```python
from build123d import *
from build123d.topology import SkipClean

# Parameters (mm, degrees)
SKETCH3_R                = 15.9
BOSS_EXTRUDE1_DEPTH      = 35
SKETCH4_R                = 5
BOSS_EXTRUDE2_DEPTH      = 32.5
SKETCH7_W                = 4.2
SKETCH7_H                = 5.15
SKETCH7_W_2              = 5.6
SKETCH7_H_2              = 2.4
BOSS_EXTRUDE3_DEPTH      = 5
BOSS_EXTRUDE3_DEPTH_BACK = 5
SKETCH8_R                = 6.25
SKETCH8_R_2              = 3
SKETCH9_R                = 3
CUT_EXTRUDE1_DEPTH       = 16


with BuildPart() as part:
    # Sketch3 → Boss-Extrude1 (new body)
    with BuildSketch(Plane.XY):
        Circle(SKETCH3_R)
    extrude(amount=BOSS_EXTRUDE1_DEPTH)

    # Sketch4 → Boss-Extrude2 (add)
    with BuildSketch(Plane.XY.offset(35)):
        Circle(SKETCH4_R)
    extrude(amount=BOSS_EXTRUDE2_DEPTH)

    # Sketch7 → Cut-Revolve1 (revolve, cut)
    with BuildSketch(Plane(origin=(0, 0, 0), x_dir=(0, 0, -1), z_dir=(1, 0, 0)), mode=Mode.PRIVATE) as cut_revolve1_sk:
        with Locations((-17.5, 13.325)):
            Rectangle(SKETCH7_W, SKETCH7_H)
        with Locations((-27.4, 14.7)):
            Rectangle(SKETCH7_W_2, SKETCH7_H_2)
        with Locations((-7.6, 14.7)):
            Rectangle(SKETCH7_W_2, SKETCH7_H_2)
    revolve(cut_revolve1_sk.sketch.rotate(Axis((0, 0, -11.998492927), (0, 0, 1)), 90), axis=Axis((0, 0, -11.998492927), (0, 0, 1)), mode=Mode.SUBTRACT)

    # Sketch8 → Boss-Extrude3 (add, two sides: drawn at the far end of the back side and taken through both)
    with SkipClean():  # the faces are left unmerged after this step: merging them gives an invalid solid
        with BuildSketch(Plane(origin=(0, 0, 0), x_dir=(1, 0, 0), z_dir=(0, 1, 0)).offset(-BOSS_EXTRUDE3_DEPTH_BACK)):
            with Locations((0, -67.5)):
                Circle(SKETCH8_R)
            with Locations(Location((0, -67.5, 0), (0, 0, 270))):
                Circle(SKETCH8_R_2, mode=Mode.SUBTRACT)
        extrude(amount=BOSS_EXTRUDE3_DEPTH + BOSS_EXTRUDE3_DEPTH_BACK)

    # Sketch9 → Cut-Extrude1 (cut)
    with SkipClean():  # the faces are left unmerged after this step: merging them gives an invalid solid
        with BuildSketch(Plane(origin=(0, 5, 0), x_dir=(1, 0, 0), z_dir=(0, 1, 0))):
            with Locations(Location((0, -67.5, 0), (0, 0, 270))):
                Circle(SKETCH9_R)
        extrude(amount=-CUT_EXTRUDE1_DEPTH, mode=Mode.SUBTRACT)


solid = part.part
```
Read the model definition and answer for the solid it produces. Units are mm, in the model's axes. A direction names the side the tool comes from. Round coordinates to 2 decimals unless told otherwise and drop trailing zeros. Loops run counter-clockwise (first coordinate to the right, second up) from the corner with the lowest first, then second, coordinate; pieces in that order, holes last. Notation, with made-up numbers: (-36.75, 80.5) -> (11.25, 80.5) arc R15 cw to (11.25, 101.5) -> close; hole circle Ø5 at (22, -1.75). An arc over 180 degrees is marked (long way). One line per item, written item: value.
1) A cutting plane is placed at D-D (x = -7). Determine the outline of the cut face in (y, z).
Answer list:
outline: (-14.28, 0) -> (14.28, 0) -> (14.28, 4.8) -> (11.54, 4.8) -> (11.54, 10.4) -> (14.28, 10.4) -> (14.28, 15.4) -> (8.16, 15.4) -> (8.16, 19.6) -> (14.28, 19.6) -> (14.28, 24.6) -> (11.54, 24.6) -> (11.54, 30.2) -> (14.28, 30.2) -> (14.28, 35) -> (-14.28, 35) -> (-14.28, 30.2) -> (-11.54, 30.2) -> (-11.54, 24.6) -> (-14.28, 24.6) -> (-14.28, 19.6) -> (-8.16, 19.6) -> (-8.16, 15.4) -> (-14.28, 15.4) -> (-14.28, 10.4) -> (-11.54, 10.4) -> (-11.54, 4.8) -> (-14.28, 4.8) -> close
2) For faces 4 (the face through (-7, 12, 30.2)), 5 (the face through (3, 5, 66)), 6 (the face through (3, -5, 66)), determine the directions among +Z, -Z, +X, -X, +Y, -Y from which every point of the face is accessible in a straight line to the end or side of a thin tool.
Answer list:
face 4: none
face 5: +Z, +X, -X, +Y
face 6: +Z, +X, -X, -Y
3) The mould has two halves that part along Z. Classify faces 1 (the face through (-3.45, -15.52, 32.57)), 2 (the face through (2.93, 13.18, 27.36)), 3 (the face through (0, 0, 0)): pulls with the +Z half, pulls with the -Z half, needs draft (parallel to the pull), parting line crosses it, or undercut.
Answer list:
face 1: needs draft
face 2: undercut
face 3: pulls with the -Z half
4) A cutting plane is placed at B-B (z = 66). Determine the outline of the cut face in (x, y), and give its area (3 significant figures).
Answer list:
outline: (-6.07, -5) -> (-2.6, -5) -> (-2.6, 5) -> (-6.07, 5) -> close; (2.6, -5) -> (6.07, -5) -> (6.07, 5) -> (2.6, 5) -> close
area: 69.4 mm²
5) Flat-ended cylindrical pins translate along their axes: P1, Ø14, axis at x = 2.5, z = 68, coming from the -Y side; P2, Ø10, axis at y = -1.5, z = 55.5, coming from the +X side; P3, Ø1, axis at x = 8.5, z = 29, coming from the -Y side. Find the tip coordinate at first contact, or state that the pin passes through.
Answer list:
P1: stops at y = -5
P2: stops at x = 5
P3: stops at y = -10.87
6) A cutting plane is placed at A-A (y = 14.5). Determine the outline of the cut face in (x, z).
Answer list:
outline: (-6.52, 0) -> (6.52, 0) -> (6.52, 4.8) -> (-6.52, 4.8) -> close; (-6.52, 10.4) -> (6.52, 10.4) -> (6.52, 15.4) -> (-6.52, 15.4) -> close; (-6.52, 19.6) -> (6.52, 19.6) -> (6.52, 24.6) -> (-6.52, 24.6) -> close; (-6.52, 30.2) -> (6.52, 30.2) -> (6.52, 35) -> (-6.52, 35) -> close
7) Consider L1, parallel to Z at x = 7, y = -13.5; L2, parallel to Z at x = 10, y = -9; L3, parallel to Z at x = -1, y = -7. Determine where each line is inside the solid, lowest interval first. Write a range as [from, to].
Answer list:
L1: z = [0, 4.8], [10.4, 15.4], [19.6, 24.6], [30.2, 35]
L2: z = [0, 15.4], [19.6, 35]
L3: z = [0, 35]
